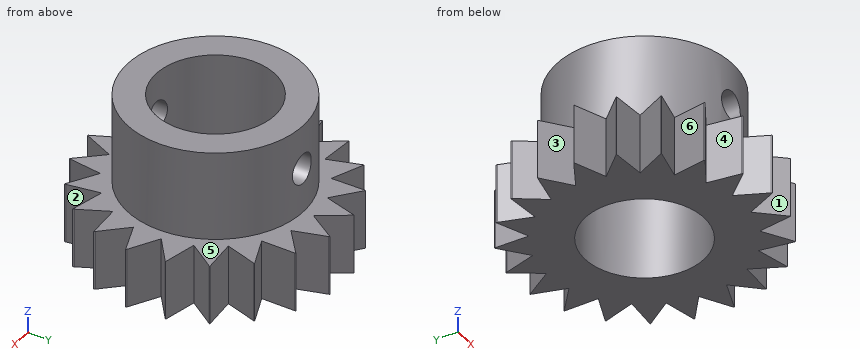
from build123d import *

# Parameters (mm, degrees)
CUT_EXTRUDE5_DEPTH      = 11.799302202
CUT_EXTRUDE5_DEPTH_BACK = 11.799302202
FILLET1_R               = 0.254
CUT_EXTRUDE4_DEPTH      = 13.513900808
CUT_EXTRUDE4_DEPTH_BACK = 13.513900808
SKETCH4_R               = 0.8001


with BuildPart() as part:
    # Sketch2 → Revolve1 (revolve)
    with BuildSketch(Plane(origin=(0, 0, 0), x_dir=(0, 0, -1), z_dir=(1, 0, 0)), mode=Mode.PRIVATE) as revolve1_sk:
        Polygon((0, 3.175), (0, 6.858), (-3.175, 6.858), (-3.175, 4.699), (-7.9248, 4.699), (-7.9248, 3.175), align=None)
    revolve(revolve1_sk.sketch.rotate(Axis((0, 0, -6.785443847), (0, 0, 1)), 90), axis=Axis((0, 0, -6.785443847), (0, 0, 1)))

    # Sketch5 → Cut-Extrude5 (cut, two sides: drawn at the far end of the back side and taken through both)
    with BuildSketch(Plane.XY.offset(3.175).offset(-CUT_EXTRUDE5_DEPTH_BACK)):
        with BuildLine():
            Line((-1.549763756, 5.024210698), (-1.028262887, 6.780474868))
            ThreePointArc((-1.028262887, 6.780474868), (-2.021430986, 6.553318302), (-2.969986829, 6.181532354))
            Line((-2.969986829, 6.181532354), (-1.549763756, 5.024210698))
        make_face()
        with BuildLine():
            Line((-2.961824201, 4.344198228), (-2.981160105, 6.176151587))
            ThreePointArc((-2.981160105, 6.176151587), (-3.863248958, 5.666345514), (-4.660077294, 5.031485229))
            Line((-4.660077294, 5.031485229), (-2.961824201, 4.344198228))
        make_face()
        with BuildLine():
            Line((-4.110713569, 3.27818468), (-4.669168164, 5.023050135))
            ThreePointArc((-4.669168164, 5.023050135), (-5.361800307, 4.275893061), (-5.936099441, 3.434368562))
            Line((-5.936099441, 3.434368562), (-4.110713569, 3.27818468))
        make_face()
        with BuildLine():
            Line((-4.894347996, 1.920890038), (-5.942300142, 3.423628634))
            ThreePointArc((-5.942300142, 3.423628634), (-6.383932168, 2.505508745), (-6.684673103, 1.532093177))
            Line((-6.684673103, 1.532093177), (-4.894347996, 1.920890038))
        make_face()
        with BuildLine():
            Line((-5.243098125, 0.392915886), (-6.687432674, 1.520002705))
            ThreePointArc((-6.687432674, 1.520002705), (-6.838823641, 0.512498982), (-6.839284225, -0.50631541))
            Line((-6.839284225, -0.50631541), (-5.243098125, 0.392915886))
        make_face()
        with BuildLine():
            Line((-5.125975977, -1.169970567), (-6.838357467, -0.518682134))
            ThreePointArc((-6.838357467, -0.518682134), (-6.686055622, -1.526048565), (-6.386194929, -2.499735652))
            Line((-6.386194929, -2.499735652), (-5.125975977, -1.169970567))
        make_face()
        with BuildLine():
            Line((-4.553388368, -2.6289), (-6.381664189, -2.51127979))
            ThreePointArc((-6.381664189, -2.51127979), (-5.939202219, -3.429), (-5.365664189, -4.271043411))
            Line((-5.365664189, -4.271043411), (-4.553388368, -2.6289))
        make_face()
        with BuildLine():
            Line((-3.576212221, -3.854240132), (-5.357932042, -4.280739216))
            ThreePointArc((-5.357932042, -4.280739216), (-4.664624636, -5.027269737), (-3.868370638, -5.662850219))
            Line((-3.868370638, -5.662850219), (-3.576212221, -3.854240132))
        make_face()
        with BuildLine():
            Line((-2.281273924, -4.737114114), (-3.85812412, -5.669836177))
            ThreePointArc((-3.85812412, -5.669836177), (-2.975574683, -6.178844496), (-2.02735538, -6.551487935))
            Line((-2.02735538, -6.551487935), (-2.281273924, -4.737114114))
        make_face()
        with BuildLine():
            Line((-0.783634427, -5.199074718), (-2.015504939, -6.555143312))
            ThreePointArc((-2.015504939, -6.555143312), (-1.022131861, -6.781401806), (-0.0062007, -6.857997197))
            Line((-0.0062007, -6.857997197), (-0.783634427, -5.199074718))
        make_face()
        with BuildLine():
            ThreePointArc((0.0062007, -6.857997197), (1.022131861, -6.781401806), (2.015504939, -6.555143312))
            Line((2.015504939, -6.555143312), (0.783634427, -5.199074718))
            Line((0.783634427, -5.199074718), (0.0062007, -6.857997197))
        make_face()
        with BuildLine():
            ThreePointArc((2.02735538, -6.551487935), (2.975574683, -6.178844496), (3.85812412, -5.669836177))
            Line((3.85812412, -5.669836177), (2.281273924, -4.737114114))
            Line((2.281273924, -4.737114114), (2.02735538, -6.551487935))
        make_face()
        with BuildLine():
            ThreePointArc((3.868370638, -5.662850219), (4.664624636, -5.027269737), (5.357932042, -4.280739216))
            Line((5.357932042, -4.280739216), (3.576212221, -3.854240132))
            Line((3.576212221, -3.854240132), (3.868370638, -5.662850219))
        make_face()
        with BuildLine():
            ThreePointArc((5.365664189, -4.271043411), (5.939202219, -3.429), (6.381664189, -2.51127979))
            Line((6.381664189, -2.51127979), (4.553388368, -2.6289))
            Line((4.553388368, -2.6289), (5.365664189, -4.271043411))
        make_face()
        with BuildLine():
            ThreePointArc((6.386194929, -2.499735652), (6.686055622, -1.526048565), (6.838357467, -0.518682134))
            Line((6.838357467, -0.518682134), (5.125975977, -1.169970567))
            Line((5.125975977, -1.169970567), (6.386194929, -2.499735652))
        make_face()
        with BuildLine():
            ThreePointArc((6.858, 0), (6.815224768, 0.764771443), (6.687432674, 1.520002705))
            Line((6.687432674, 1.520002705), (5.243098125, 0.392915886))
            Line((5.243098125, 0.392915886), (6.839284225, -0.50631541))
            ThreePointArc((6.839284225, -0.50631541), (6.853319459, -0.253330602), (6.858, 0))
        make_face()
        with BuildLine():
            ThreePointArc((6.684673103, 1.532093177), (6.383932168, 2.505508745), (5.942300142, 3.423628634))
            Line((5.942300142, 3.423628634), (4.894347996, 1.920890038))
            Line((4.894347996, 1.920890038), (6.684673103, 1.532093177))
        make_face()
        with BuildLine():
            ThreePointArc((5.936099441, 3.434368562), (5.361800307, 4.275893061), (4.669168164, 5.023050135))
            Line((4.669168164, 5.023050135), (4.110713569, 3.27818468))
            Line((4.110713569, 3.27818468), (5.936099441, 3.434368562))
        make_face()
        with BuildLine():
            ThreePointArc((4.660077294, 5.031485229), (3.863248958, 5.666345514), (2.981160105, 6.176151587))
            Line((2.981160105, 6.176151587), (2.961824201, 4.344198228))
            Line((2.961824201, 4.344198228), (4.660077294, 5.031485229))
        make_face()
        with BuildLine():
            ThreePointArc((2.969986829, 6.181532354), (2.021430986, 6.553318302), (1.028262887, 6.780474868))
            Line((1.028262887, 6.780474868), (1.549763756, 5.024210698))
            Line((1.549763756, 5.024210698), (2.969986829, 6.181532354))
        make_face()
        with BuildLine():
            Line((0, 6.858), (0, 5.2578))
            Line((0, 5.2578), (1.016, 6.782323201))
            ThreePointArc((1.016, 6.782323201), (0.509407248, 6.839054632), (0, 6.858))
        make_face()
        with BuildLine():
            Line((-1.016, 6.782323201), (0, 5.2578))
            Line((0, 5.2578), (0, 6.858))
            ThreePointArc((0, 6.858), (-0.509407248, 6.839054632), (-1.016, 6.782323201))
        make_face()
    extrude(amount=CUT_EXTRUDE5_DEPTH + CUT_EXTRUDE5_DEPTH_BACK, mode=Mode.SUBTRACT)

    # Fillet1
    # the kernel refuses this fillet: 0.254 mm, written as the material it takes off along each edge
    with BuildSketch(Plane(origin=(1.028262887, 6.780474868, -0.173566316), x_dir=(0.2846534382375399, -0.958630491951694, 0), z_dir=(0, 0, 1)), Plane(origin=(2.981160105, 6.176151587, -0.173566316), x_dir=(-0.010554213197513457, -0.9999443027407983, 0), z_dir=(0, 0, 1)), Plane(origin=(4.669168164, 5.023050135, -0.173566316), x_dir=(-0.3048240764735684, -0.9524086740480875, 0), z_dir=(0, 0, 1)), Plane(origin=(5.942300142, 3.423628634, -0.173566316), x_dir=(-0.5720089828565192, -0.8202473550895794, 0), z_dir=(0, 0, 1))) as fillet1_piece_1:
        with BuildLine():
            CenterArc((0.069426526, -0.254), FILLET1_R, 90, 17.100666737)
            Line((-0.005262541, -0.011229443), (-0.006756323, -0.006374032))
            ThreePointArc((-0.006756323, -0.006374032), (-0.007233739, -0.003457831), (-0.004597979, 0.002159859))
            Line((-0.004597979, 0.002159859), (0, 0.00508))
            Line((0, 0.00508), (0.069426526, 0.00508))
            Line((0.069426526, 0.00508), (0.069426526, 0))
        make_face()
    extrude(amount=3.522132632, mode=Mode.SUBTRACT)
    with BuildSketch(Plane(origin=(6.687432674, 1.520002705, 3.348566316), x_dir=(-0.7883683808925953, -0.6152034590351292, 0), z_dir=(0, 0, -1)), Plane(origin=(-0.0062007, -6.857997197, 3.348566316), x_dir=(-0.4243505554663044, 0.9054979878914358, 0), z_dir=(0, 0, -1)), Plane(origin=(-2.02735538, -6.551487935, 3.348566316), x_dir=(-0.13859763357417676, 0.9903487749109595, 0), z_dir=(0, 0, -1)), Plane(origin=(-3.868370638, -5.662850219, 3.348566316), x_dir=(0.15947029628670847, 0.9872027272056279, 0), z_dir=(0, 0, -1)), Plane(origin=(-5.365664189, -4.271043411, 3.348566316), x_dir=(0.4433685904986441, 0.8963393849202688, 0), z_dir=(0, 0, -1)), Plane(origin=(-6.386194929, -2.499735652, 3.348566316), x_dir=(0.687871639753785, 0.7258323547641282, 0), z_dir=(0, 0, -1)), Plane(origin=(-6.684673103, 1.532093177, 3.348566316), x_dir=(0.9772221447470836, 0.21221894311279188, 0), z_dir=(0, 0, -1))) as fillet1_piece_2:
        with BuildLine():
            CenterArc((0.069426526, 0.254), FILLET1_R, 252.899333263, 17.100666737)
            Line((-0.005262541, 0.011229443), (-0.006756323, 0.006374032))
            ThreePointArc((-0.006756323, 0.006374032), (-0.007233739, 0.003457831), (-0.004597979, -0.002159859))
            Line((-0.004597979, -0.002159859), (0, -0.00508))
            Line((0, -0.00508), (0.069426526, -0.00508))
            Line((0.069426526, -0.00508), (0.069426526, 0))
        make_face()
    extrude(amount=3.522132632, mode=Mode.SUBTRACT)
    with BuildSketch(Plane(origin=(6.839284225, -0.50631541, 3.348566316), x_dir=(-0.07473009358640008, -0.9972037971811819, 0), z_dir=(0, 0, -1)), Plane(origin=(6.386194929, -2.499735652, 3.348566316), x_dir=(-0.3653410243663928, -0.9308737486442051, 0), z_dir=(0, 0, -1)), Plane(origin=(5.365664189, -4.271043411, 3.348566316), x_dir=(-0.623489801858665, -0.7818314824680845, 0), z_dir=(0, 0, -1)), Plane(origin=(3.868370638, -5.662850219, 3.348566316), x_dir=(-0.8262387743159489, -0.5633200580636893, 0), z_dir=(0, 0, -1)), Plane(origin=(2.02735538, -6.551487935, 3.348566316), x_dir=(-0.9555728057861146, -0.2947551744109893, 0), z_dir=(0, 0, -1)), Plane(origin=(-1.028262887, 6.780474868, 3.348566316), x_dir=(0.9888308262251171, 0.14904226617625063, 0), z_dir=(0, 0, -1)), Plane(origin=(-2.981160105, 6.176151587, 3.348566316), x_dir=(0.9009688679024408, 0.4338837391175129, 0), z_dir=(0, 0, -1)), Plane(origin=(-4.669168164, 5.023050135, 3.348566316), x_dir=(0.7330518718297447, 0.6801727377710072, 0), z_dir=(0, 0, -1)), Plane(origin=(-5.942300142, 3.423628634, 3.348566316), x_dir=(0.50000000000004, 0.8660254037844156, 0), z_dir=(0, 0, -1))) as fillet1_piece_3:
        with BuildLine():
            CenterArc((0.200535304, 0.170650621), FILLET1_R, 205.109562615, 17.100666737)
            Line((-0.029461185, 0.06286558), (-0.034061115, 0.060709879))
            Line((-0.034061115, 0.060709879), (-0.00459993, -0.002155701))
            Line((-0.00459993, -0.002155701), (-4.593e-06, -0.005079998))
            ThreePointArc((-4.593e-06, -0.005079998), (0.0062007, -0.005082803), (0.008638723, -0.003413012))
            Line((0.008638723, -0.003413012), (0.012401401, 0))
        make_face()
    extrude(amount=3.522132632, mode=Mode.SUBTRACT)
    with BuildSketch(Plane(origin=(-6.839284225, -0.50631541, 3.348566316), x_dir=(0.07473009358634887, -0.9972037971811858, 0), z_dir=(0, 0, -1))) as fillet1_piece_4:
        with BuildLine():
            CenterArc((0.200535304, -0.170650621), FILLET1_R, 137.789770648, 17.100666737)
            Line((-0.029461185, -0.06286558), (-0.034061115, -0.060709879))
            Line((-0.034061115, -0.060709879), (-0.00459993, 0.002155701))
            Line((-0.00459993, 0.002155701), (-4.593e-06, 0.005079998))
            ThreePointArc((-4.593e-06, 0.005079998), (0.0062007, 0.005082803), (0.008638723, 0.003413012))
            Line((0.008638723, 0.003413012), (0.012401401, 0))
        make_face()
    extrude(amount=3.522132632, mode=Mode.SUBTRACT)

    # Sketch4 → Cut-Extrude4 (cut, two sides: drawn at the far end of the back side and taken through both)
    with BuildSketch(Plane(origin=(0, 0, 0), x_dir=(1, 0, 0), z_dir=(0, 1, 0)).offset(-CUT_EXTRUDE4_DEPTH_BACK)):
        with Locations(Location((0, -5.5626, 0), (0, 0, 270))):
            Circle(SKETCH4_R)
    extrude(amount=CUT_EXTRUDE4_DEPTH + CUT_EXTRUDE4_DEPTH_BACK, mode=Mode.SUBTRACT)


solid = part.part
Design review of the part built by this model. Coordinates are the model's own, in mm. Face numbers are marked on the shaded views. A direction names the side the tool comes from. Coordinates: 2 decimals unless noted, no trailing zeros. Order: outer loops, then holes, each group sorted by start corner. A loop starts at its lowest first (then second) coordinate and runs counter-clockwise, first axis right, second up. Notation, with made-up numbers: (75, 33.5) -> (99, 33.5) arc R22 cw to (99, 56.5) -> close; hole circle Ø8 at (-17, 84.5). An arc over 180 degrees is marked (long way). One line per item, written item: value.
1) Machinability: for the marked faces 1, 2 and 3, which of the approach directions +Z, -Z, +X, -X, +Y, -Y give a long, thin tool a straight path to every point of the face, cutting with its end or side? Answer none if there is none.
Output values:
face 1: +Z, -Z, -Y
face 2: +Z, -Z
face 3: +Z, -Z, -X
2) We need section B-B, the plane x = 2.75. Give the boundary of the cut face in (y, z) (3 decimals), then the cut area to 3 significant figures.
Output values:
outline: (-5.014, 0) -> (-1.587, 0) -> (-1.587, 7.925) -> (-3.81, 7.925) -> (-3.81, 3.175) -> (-5.014, 3.175) -> close; (1.587, 0) -> (6.002, 0) -> (6.002, 3.175) -> (3.81, 3.175) -> (3.81, 7.925) -> (1.587, 7.925) -> close
area: 46.0 mm2
3) Draft analysis for pull direction Y (two halves, no side actions). For the marked faces 4, 5 and 6, state which applies: +Y half, -Y half, draft (parallel to the pull), parting line (faces both ways), or undercut.
Output values:
face 4: -Y half
face 5: draft
face 6: undercut
4) We need section C-C, the plane z = 4.5. Give the boundary of the cut face in (x, y) (3 decimals).
Output values:
outline: circle Ø9.398 at (0, 0); hole circle Ø6.35 at (0, 0)
5) We need section A-A, the plane y = 0. Give the boundary of the cut face in (x, z) (3 decimals).
Output values:
outline: (-5.941, 0) -> (-3.175, 0) -> (-3.175, 7.925) -> (-4.699, 7.925) -> (-4.699, 3.175) -> (-5.941, 3.175) -> close; (3.175, 0) -> (5.941, 0) -> (5.941, 3.175) -> (4.699, 3.175) -> (4.699, 7.925) -> (3.175, 7.925) -> close
6) To check wall thickness, follow probe 1 along Z at (x, y) = (0, 4.1); probe 2 along Z at (x, y) = (-2.75, 5.5) (3 decimals); probe 3 along Y at (x, z) = (-2.25, 6.25). State the ranges of each line that lie inside material, in increasing order. Write a range as [from, to].
Output values:
probe 1: z = [0, 4.76], [6.36, 7.92]
probe 2: z = [0, 3.175]
probe 3: y = [-4.13, -2.24], [2.24, 4.13]
7) Clearance check with flat-ended pins moving along their axes: P1, Ø1.5, axis at y = 2.5, z = 2.5, coming from the +X side; P2, Ø2, axis at y = -4, z = 3, coming from the +X side; P3, Ø2, axis at x = 0, z = 5.56, coming from the -Y side. State where each tip first meets the part, or that it passes through.
Output values:
P1: stops at x = 5.82
P2: stops at x = 5.36
P3: stops at y = -4.7
